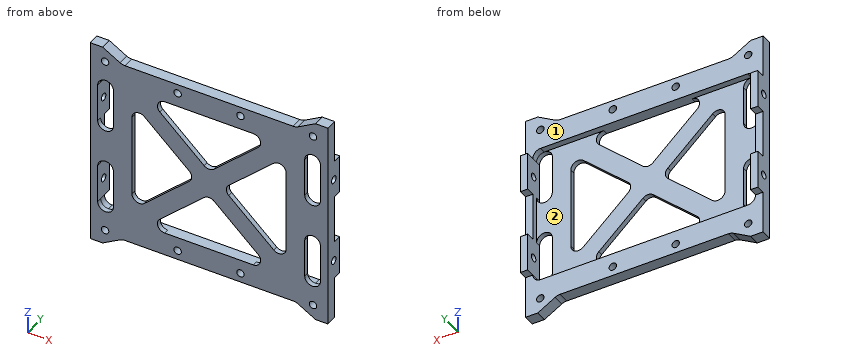
from build123d import *

# Parameters (mm, degrees)
SKETCH1_R           = 1.5
BOSS_EXTRUDE1_DEPTH = 2
SKETCH2_R           = 1.5
BOSS_EXTRUDE2_DEPTH = 2.5
BOSS_EXTRUDE3_START = -3
SKETCH3_W           = 15.5
SKETCH3_H           = 3.5
BOSS_EXTRUDE3_DEPTH = 3
SKETCH4_R           = 1.5
CUT_EXTRUDE1_DEPTH  = 5
CUT_EXTRUDE2_DEPTH  = 65.325422657


with BuildPart() as part:
    # Sketch1 → Boss-Extrude1 (new body)
    with BuildSketch(Plane(origin=(0, 0, 0), x_dir=(1, 0, 0), z_dir=(0, 1, 0))):
        with BuildLine():
            Line((-48, -42.4), (-43, -42.4))
            Line((-43, -42.4), (-36.009266938, -38.363898385))
            ThreePointArc((-36.009266938, -38.363898385), (-35.044543118, -37.964296695), (-34.009266938, -37.828))
            Line((-34.009266938, -37.828), (34.009266938, -37.828))
            ThreePointArc((34.009266938, -37.828), (35.044543118, -37.964296695), (36.009266938, -38.363898385))
            Line((36.009266938, -38.363898385), (43, -42.4))
            Line((43, -42.4), (48, -42.4))
            Line((48, -42.4), (48, 42.4))
            Line((48, 42.4), (43, 42.4))
            Line((43, 42.4), (36.009266938, 38.363898385))
            ThreePointArc((36.009266938, 38.363898385), (35.044543118, 37.964296695), (34.009266938, 37.828))
            Line((34.009266938, 37.828), (-34.009266938, 37.828))
            ThreePointArc((-34.009266938, 37.828), (-35.044543118, 37.964296695), (-36.009266938, 38.363898385))
            Line((-36.009266938, 38.363898385), (-43, 42.4))
            Line((-43, 42.4), (-48, 42.4))
            Line((-48, 42.4), (-48, -42.4))
        make_face()
        with Locations(Location((-12.7, -34.078, 0), (0, 0, 270))):
            Circle(SKETCH1_R, mode=Mode.SUBTRACT)
        with Locations(Location((12.7, -34.078, 0), (0, 0, 270))):
            Circle(SKETCH1_R, mode=Mode.SUBTRACT)
        with Locations(Location((-12.7, 34.078, 0), (0, 0, 270))):
            Circle(SKETCH1_R, mode=Mode.SUBTRACT)
        with Locations(Location((12.7, 34.078, 0), (0, 0, 270))):
            Circle(SKETCH1_R, mode=Mode.SUBTRACT)
        with Locations(Location((-42, 36.5, 0), (0, 0, 270))):
            Circle(SKETCH1_R, mode=Mode.SUBTRACT)
        with Locations(Location((42, 36.5, 0), (0, 0, 270))):
            Circle(SKETCH1_R, mode=Mode.SUBTRACT)
        with Locations(Location((42, -36.5, 0), (0, 0, 270))):
            Circle(SKETCH1_R, mode=Mode.SUBTRACT)
        with Locations(Location((-42, -36.5, 0), (0, 0, 270))):
            Circle(SKETCH1_R, mode=Mode.SUBTRACT)
        with BuildLine():
            Line((-38.65, 25.25), (-38.65, 9.75))
            ThreePointArc((-38.65, 9.75), (-41.825, 6.575), (-45, 9.75))
            Line((-45, 9.75), (-45, 25.25))
            ThreePointArc((-45, 25.25), (-41.825, 28.425), (-38.65, 25.25))
        make_face(mode=Mode.SUBTRACT)
        with BuildLine():
            Line((-38.65, -9.75), (-38.65, -25.25))
            ThreePointArc((-38.65, -25.25), (-41.825, -28.425), (-45, -25.25))
            Line((-45, -25.25), (-45, -9.75))
            ThreePointArc((-45, -9.75), (-41.825, -6.575), (-38.65, -9.75))
        make_face(mode=Mode.SUBTRACT)
        with BuildLine():
            Line((45, 25.25), (45, 9.75))
            ThreePointArc((45, 9.75), (41.825, 6.575), (38.65, 9.75))
            Line((38.65, 9.75), (38.65, 25.25))
            ThreePointArc((38.65, 25.25), (41.825, 28.425), (45, 25.25))
        make_face(mode=Mode.SUBTRACT)
        with BuildLine():
            Line((45, -9.75), (45, -25.25))
            ThreePointArc((45, -25.25), (41.825, -28.425), (38.65, -25.25))
            Line((38.65, -25.25), (38.65, -9.75))
            ThreePointArc((38.65, -9.75), (41.825, -6.575), (45, -9.75))
        make_face(mode=Mode.SUBTRACT)
    extrude(amount=BOSS_EXTRUDE1_DEPTH)

    # Sketch2 → Boss-Extrude2 (add)
    with BuildSketch(Plane(origin=(0, 2, 0), x_dir=(1, 0, 0), z_dir=(0, 1, 0))):
        with BuildLine():
            Line((48, -42.4), (48, 42.4))
            Line((48, 42.4), (43, 42.4))
            Line((43, 42.4), (36.009266938, 38.363898385))
            ThreePointArc((36.009266938, 38.363898385), (35.044543118, 37.964296695), (34.009266938, 37.828))
            Line((34.009266938, 37.828), (-34.009266938, 37.828))
            ThreePointArc((-34.009266938, 37.828), (-35.044543118, 37.964296695), (-36.009266938, 38.363898385))
            Line((-36.009266938, 38.363898385), (-43, 42.4))
            Line((-43, 42.4), (-48, 42.4))
            Line((-48, 42.4), (-48, -42.4))
            Line((-48, -42.4), (-43, -42.4))
            Line((-43, -42.4), (-36.009266938, -38.363898385))
            ThreePointArc((-36.009266938, -38.363898385), (-35.044543118, -37.964296695), (-34.009266938, -37.828))
            Line((-34.009266938, -37.828), (34.009266938, -37.828))
            ThreePointArc((34.009266938, -37.828), (35.044543118, -37.964296695), (36.009266938, -38.363898385))
            Line((36.009266938, -38.363898385), (43, -42.4))
            Line((43, -42.4), (48, -42.4))
        make_face()
        with Locations((-42, -36.5)):
            Circle(SKETCH2_R, mode=Mode.SUBTRACT)
        with Locations((-12.7, -34.078)):
            Circle(SKETCH2_R, mode=Mode.SUBTRACT)
        with Locations((12.7, -34.078)):
            Circle(SKETCH2_R, mode=Mode.SUBTRACT)
        with Locations((42, -36.5)):
            Circle(SKETCH2_R, mode=Mode.SUBTRACT)
        with Locations((-42, 36.5)):
            Circle(SKETCH2_R, mode=Mode.SUBTRACT)
        with Locations((-12.7, 34.078)):
            Circle(SKETCH2_R, mode=Mode.SUBTRACT)
        with BuildLine():
            Line((45, 9.75), (45, -9.75))
            Line((45, -9.75), (45, -25.25))
            ThreePointArc((45, -25.25), (44.07006403, -27.49506403), (41.825, -28.425))
            Line((41.825, -28.425), (-41.825, -28.425))
            ThreePointArc((-41.825, -28.425), (-44.07006403, -27.49506403), (-45, -25.25))
            Line((-45, -25.25), (-45, -9.75))
            Line((-45, -9.75), (-45, 9.75))
            Line((-45, 9.75), (-45, 25.25))
            ThreePointArc((-45, 25.25), (-44.07006403, 27.49506403), (-41.825, 28.425))
            Line((-41.825, 28.425), (41.825, 28.425))
            ThreePointArc((41.825, 28.425), (44.07006403, 27.49506403), (45, 25.25))
            Line((45, 25.25), (45, 9.75))
        make_face(mode=Mode.SUBTRACT)
        with Locations((12.7, 34.078)):
            Circle(SKETCH2_R, mode=Mode.SUBTRACT)
        with Locations((42, 36.5)):
            Circle(SKETCH2_R, mode=Mode.SUBTRACT)
    extrude(amount=BOSS_EXTRUDE2_DEPTH)

    # Sketch3 → Boss-Extrude3 (add)
    with BuildSketch(Plane(origin=(48, 0, 0), x_dir=(0, 0, -1), z_dir=(1, 0, 0)).offset(BOSS_EXTRUDE3_START)):
        with Locations((-17.5, 6.25)):
            Rectangle(SKETCH3_W, SKETCH3_H)
        with Locations((17.5, 6.25)):
            Rectangle(SKETCH3_W, SKETCH3_H)
    boss_extrude3 = extrude(amount=BOSS_EXTRUDE3_DEPTH)

    # Sketch4 → Cut-Extrude1 (cut)
    with BuildSketch(Plane(origin=(48, 0, 0), x_dir=(0, 0, -1), z_dir=(1, 0, 0))):
        with Locations((-17.5, 4)):
            Circle(SKETCH4_R)
        with Locations((17.5, 4)):
            Circle(SKETCH4_R)
    cut_extrude1 = extrude(amount=-CUT_EXTRUDE1_DEPTH, mode=Mode.SUBTRACT)

    # Mirror1: Boss-Extrude3, Cut-Extrude1 across plane
    add(boss_extrude3.mirror(Plane(origin=(0, 0, 0), x_dir=(0, 0, 1), z_dir=(1, 0, 0))))
    add(cut_extrude1.mirror(Plane(origin=(0, 0, 0), x_dir=(0, 0, 1), z_dir=(1, 0, 0))), mode=Mode.SUBTRACT)

    # Sketch5 → Cut-Extrude2 (cut, through all)
    with BuildSketch(Plane(origin=(0, 2, 0), x_dir=(1, 0, 0), z_dir=(0, 1, 0))):
        with BuildLine():
            Line((-26.127824556, -18.76552712), (-7.991792465, -2.216033952))
            ThreePointArc((-7.991792465, -2.216033952), (-7.013967909, 0), (-7.991792465, 2.216033952))
            Line((-7.991792465, 2.216033952), (-26.127824556, 18.76552712))
            ThreePointArc((-26.127824556, 18.76552712), (-29.361089111, 19.294172233), (-31.15, 16.549493168))
            Line((-31.15, 16.549493168), (-31.15, -16.549493168))
            ThreePointArc((-31.15, -16.549493168), (-29.361089111, -19.294172233), (-26.127824556, -18.76552712))
        make_face()
        with BuildLine():
            Line((19.87060859, 23.208966048), (2.022175444, 6.921912688))
            ThreePointArc((2.022175444, 6.921912688), (0, 6.137946639), (-2.022175444, 6.921912688))
            Line((-2.022175444, 6.921912688), (-19.87060859, 23.208966048))
            ThreePointArc((-19.87060859, 23.208966048), (-20.645583648, 26.509411856), (-17.848433147, 28.425))
            Line((-17.848433147, 28.425), (17.848433147, 28.425))
            ThreePointArc((17.848433147, 28.425), (20.645583648, 26.509411856), (19.87060859, 23.208966048))
        make_face()
        with BuildLine():
            Line((-19.87060859, -23.208966048), (-2.022175444, -6.921912688))
            ThreePointArc((-2.022175444, -6.921912688), (0, -6.137946639), (2.022175444, -6.921912688))
            Line((2.022175444, -6.921912688), (19.87060859, -23.208966048))
            ThreePointArc((19.87060859, -23.208966048), (20.645583648, -26.509411856), (17.848433147, -28.425))
            Line((17.848433147, -28.425), (-17.848433147, -28.425))
            ThreePointArc((-17.848433147, -28.425), (-20.645583648, -26.509411856), (-19.87060859, -23.208966048))
        make_face()
        with BuildLine():
            Line((7.991792465, 2.216033952), (26.127824556, 18.76552712))
            ThreePointArc((26.127824556, 18.76552712), (29.361089111, 19.294172233), (31.15, 16.549493168))
            Line((31.15, 16.549493168), (31.15, -16.549493168))
            ThreePointArc((31.15, -16.549493168), (29.361089111, -19.294172233), (26.127824556, -18.76552712))
            Line((26.127824556, -18.76552712), (7.991792465, -2.216033952))
            ThreePointArc((7.991792465, -2.216033952), (7.013967909, 0), (7.991792465, 2.216033952))
        make_face()
    extrude(amount=-CUT_EXTRUDE2_DEPTH, mode=Mode.SUBTRACT)


solid = part.part
Work out the finished part from the listing and answer in its coordinate system (mm). Face numbers are marked on the shaded views. Give positions to 0.01 mm unless a question says otherwise; leave off trailing zeros. Write each loop counter-clockwise with the first axis right and the second up, starting at its lowest first coordinate (ties: lowest second). Pieces come first, ordered by that corner, then holes.
Q1. Given pin 1 (17 mm diameter, centred on x = -5.5, z = -5, fed in from +Y); pin 2 (1.5 mm diameter, centred on x = -46.5, y = 5.5, fed in from +Z); pin 3 (1.3 mm diameter, centred on x = 5, y = 2, fed in from -Z); pin 4 (2.5 mm diameter, centred on x = -42, z = -36.5, fed in from +Y), each flat-ended and moving along its own axis, determine where each tip first touches the part or whether it passes through.
Answer:
pin 1: stops at y = 2
pin 2: stops at z = 25.25
pin 3: stops at z = -37.83
pin 4: passes through
Q2. The part is cut by section C-C on z = 12. Give the vertices of the cut face in (x, y), and give its area (3 significant figures).
Answer:
outline: (-48, 0) - (-45, 0) - (-45, 8) - (-48, 8) - close; (-38.65, 0) - (-31.15, 0) - (-31.15, 2) - (-38.65, 2) - close; (-18.71, 0) - (-7.59, 0) - (-7.59, 2) - (-18.71, 2) - close; (7.59, 0) - (18.71, 0) - (18.71, 2) - (7.59, 2) - close; (31.15, 0) - (38.65, 0) - (38.65, 2) - (31.15, 2) - close; (45, 0) - (48, 0) - (48, 8) - (45, 8) - close
area: 123 mm2
Q3. Straight lines are drawn through the part: L1, parallel to Z at x = -45.75, y = 4; L2, parallel to Z at x = 42, y = 2.15; L3, parallel to Z at x = -42, y = 1.25. For each, find the intervals that lie inside material, in ascending order.
Answer:
L1: z = -42.4 to -19, -16 to 16, 19 to 42.4
L2: z = -41.82 to -38, -35 to -28.42, 28.42 to 35, 38 to 41.82
L3: z = -41.82 to -38, -35 to -28.42, -6.58 to 6.58, 28.42 to 35, 38 to 41.82
Q4. The part is cut by section B-B on z = 0.5. Give the vertices of the cut face in (x, y).
Answer:
outline: (-48, 0) - (-31.15, 0) - (-31.15, 2) - (-45, 2) - (-45, 4.5) - (-48, 4.5) - close; (-7.06, 0) - (7.06, 0) - (7.06, 2) - (-7.06, 2) - close; (31.15, 0) - (48, 0) - (48, 4.5) - (45, 4.5) - (45, 2) - (31.15, 2) - close
Q5. The part is cut by section D-D on z = 30. Give the vertices of the cut face in (x, y), and give its area (3 significant figures).
Answer:
outline: (-48, 0) - (48, 0) - (48, 4.5) - (-48, 4.5) - close
area: 432 mm2
Q6. The part is cut by section A-A on x = -10. Give the vertices of the cut face in (y, z) (3 decimals), and give its area (3 significant figures).
Answer:
outline: (0, -37.828) - (4.5, -37.828) - (4.5, -28.425) - (0, -28.425) - close; (0, -14.202) - (2, -14.202) - (2, -4.049) - (0, -4.049) - close; (0, 4.049) - (2, 4.049) - (2, 14.202) - (0, 14.202) - close; (0, 28.425) - (4.5, 28.425) - (4.5, 37.828) - (0, 37.828) - close
area: 125 mm2
Q7. For a pull along Z with two mould halves and no side action, classify the marked faces 1 and 2 as released by +Z, released by -Z, zero draft, split by the parting line, or undercut.
Answer:
face 1: zero draft
face 2: undercut
